```python
from build123d import *

# Parameters (mm, degrees)
SKETCH1_R           = 2.1
SKETCH1_R_2         = 8
SKETCH1_R_3         = 11.176
SKETCH1_R_4         = 1.75
SKETCH1_R_5         = 2.032
BOSS_EXTRUDE1_DEPTH = 5
FILLET1_R           = 5
SKETCH8_R           = 1.65
CUT_EXTRUDE3_DEPTH  = 10
SKETCH9_R           = 3.5
SKETCH9_R_2         = 1.65
CUT_EXTRUDE4_DEPTH  = 3.5


with BuildPart() as part:
    # Sketch1 → Boss-Extrude1 (new body)
    with BuildSketch(Plane(origin=(0, 0, 0), x_dir=(1, 0, 0), z_dir=(0, 1, 0))):
        with BuildLine():
            Line((67.5, -41.5), (33.05, -41.5))
            ThreePointArc((33.05, -41.5), (22.55, -31), (12.05, -41.5))
            Line((12.05, -41.5), (-67.5, -41.5))
            Line((-67.5, -41.5), (-67.5, 41.5))
            Line((-67.5, 41.5), (12.05, 41.5))
            ThreePointArc((12.05, 41.5), (22.55, 31), (33.05, 41.5))
            Line((33.05, 41.5), (67.5, 41.5))
            Line((67.5, 41.5), (67.5, -41.5))
        make_face()
        with Locations((-6.45, 29)):
            Circle(SKETCH1_R, mode=Mode.SUBTRACT)
        with Locations((51.55, 29)):
            Circle(SKETCH1_R, mode=Mode.SUBTRACT)
        with Locations((51.55, -29)):
            Circle(SKETCH1_R, mode=Mode.SUBTRACT)
        with Locations((-6.45, -29)):
            Circle(SKETCH1_R, mode=Mode.SUBTRACT)
        with Locations((22.55, 0)):
            Circle(SKETCH1_R_2, mode=Mode.SUBTRACT)
        with Locations((-35.78, 0)):
            Circle(SKETCH1_R_3, mode=Mode.SUBTRACT)
        with Locations((-62.5, 36.5)):
            Circle(SKETCH1_R_4, mode=Mode.SUBTRACT)
        with Locations((62.5, 36.5)):
            Circle(SKETCH1_R_4, mode=Mode.SUBTRACT)
        with Locations((62.5, -36.5)):
            Circle(SKETCH1_R_4, mode=Mode.SUBTRACT)
        with Locations((-62.5, -36.5)):
            Circle(SKETCH1_R_4, mode=Mode.SUBTRACT)
        with Locations((-20.413, 15.367)):
            Circle(SKETCH1_R_5, mode=Mode.SUBTRACT)
        with Locations((-20.413, -15.367)):
            Circle(SKETCH1_R_5, mode=Mode.SUBTRACT)
        with Locations((-51.147, -15.367)):
            Circle(SKETCH1_R_5, mode=Mode.SUBTRACT)
        with Locations((-51.147, 15.367)):
            Circle(SKETCH1_R_5, mode=Mode.SUBTRACT)
    extrude(amount=BOSS_EXTRUDE1_DEPTH)

    # Fillet1
    fillet1_edges = [part.edges().sort_by_distance(p)[0] for p in [
        (67.5, 2.5, -41.5),
        (67.5, 2.5, 41.5),
        (-67.5, 2.5, 41.5),
        (-67.5, 2.5, -41.5),
    ]]
    fillet(fillet1_edges, radius=FILLET1_R)

    # Sketch8 → Cut-Extrude3 (cut)
    with BuildSketch(Plane(origin=(0, 5, 0), x_dir=(1, 0, 0), z_dir=(0, 1, 0))):
        with Locations((43.1993197, 1.68214862)):
            Circle(SKETCH8_R)
        with Locations((2.921522344, 4.384015291)):
            Circle(SKETCH8_R)
        with Locations((8.6993197, -25.31785138)):
            Circle(SKETCH8_R)
    extrude(amount=-CUT_EXTRUDE3_DEPTH, mode=Mode.SUBTRACT)

    # Sketch9 → Cut-Extrude4 (cut)
    with BuildSketch(Plane(origin=(0, 5, 0), x_dir=(1, 0, 0), z_dir=(0, 1, 0))):
        with Locations((2.921522344, 4.384015291)):
            Circle(SKETCH9_R)
        with Locations((2.921522344, 4.384015291)):
            Circle(SKETCH9_R_2, mode=Mode.SUBTRACT)
        with Locations((8.6993197, -25.31785138)):
            Circle(SKETCH9_R)
        with Locations((8.6993197, -25.31785138)):
            Circle(SKETCH9_R_2, mode=Mode.SUBTRACT)
        with Locations((43.1993197, 1.68214862)):
            Circle(SKETCH9_R)
        with Locations((43.1993197, 1.68214862)):
            Circle(SKETCH9_R_2, mode=Mode.SUBTRACT)
    extrude(amount=-CUT_EXTRUDE4_DEPTH, mode=Mode.SUBTRACT)


solid = part.part
```
Build history of the part. All positions in model axes, mm. A direction names the side the tool comes from. Round coordinates to 2 decimals unless told otherwise and drop trailing zeros. Write each loop counter-clockwise with the first axis right and the second up, starting at its lowest first coordinate (ties: lowest second). Pieces come first, ordered by that corner, then holes.
1) Mould opens along X. For faces 3 (the cylindrical face through (22.781, 2.465, 31.003)), 4 (the cylindrical face through (44.724, 0.761, -1.05)), 5 (the cylindrical face through (-66, 2.54, 40.07)), 6 (the flat face through (1, 0, -1)) say: +X half, -X half, draft (parallel to the pull), parting line (faces both ways), or undercut.
2) Band-saw the part on D-D, the plane y = 3.2. Give the number of separate pieces and of enclosed holes in the cut face, and give its area (3 significant figures).
3) Band-saw the part on A-A, the plane z = -29. List the corners of the cut face in (x, y).
4) Drill centre lines: probe 1 along Z at (x, y) = (-20.5, 0.5); probe 2 along X at (y, z) = (2.05, 15.5); probe 3 along X at (y, z) = (2.95, -5.5). Where is each one in solid material? Low to high.
5) Band-saw the part on C-C, the plane x = 20. List the corners of the cut face in (y, z).
6) Band-saw the part on B-B, the plane x = 51.55. List the corners of the cut face in (y, z).
7) Pin check, flat tip, straight feed: pin 1 (5.5 mm diameter, centred on x = 2.92, z = -4.38, fed in from +Y). Stop position of the tip, or through.
8) 3-axis set-ups, long thin cutter, end or side, ignore diameter. For faces 1 (the cylindrical face through (39.7, 3.3, -1.8)), 2 (the flat face through (48, 2, 41.5)): which of +Z, -Z, +X, -X, +Y, -Y reach the whole face in a straight line?
Ans:
1. face 3: undercut
1. face 4: undercut
1. face 5: -X half
1. face 6: draft
2. separate pieces: 1
2. enclosed holes: 17
2. area: 9,980 mm2
3. outline: (-67.5, 0) - (-8.55, 0) - (-8.55, 5) - (-67.5, 5) - close; (-4.35, 0) - (49.45, 0) - (49.45, 5) - (-4.35, 5) - close; (53.65, 0) - (67.5, 0) - (67.5, 5) - (53.65, 5) - close
4. probe 1: z = -41.5 to -17.4, -13.34 to 13.34, 17.4 to 41.5
4. probe 2: x = -67.5 to -53.17, -49.12 to -22.44, -18.39 to 67.5
4. probe 3: x = -67.5 to -45.51, -26.05 to -0.4, 6.24 to 16.74, 28.36 to 67.5
5. outline: (0, -31.31) - (5, -31.31) - (5, -7.58) - (0, -7.58) - close; (0, 7.58) - (5, 7.58) - (5, 31.31) - (0, 31.31) - close
6. outline: (0, -41.5) - (5, -41.5) - (5, -31.1) - (0, -31.1) - close; (0, -26.9) - (5, -26.9) - (5, 26.9) - (0, 26.9) - close; (0, 31.1) - (5, 31.1) - (5, 41.5) - (0, 41.5) - close
7. pin 1: stops at y = 1.5
8. face 1: +Y
8. face 2: +Z, +X, -X, +Y, -Y
